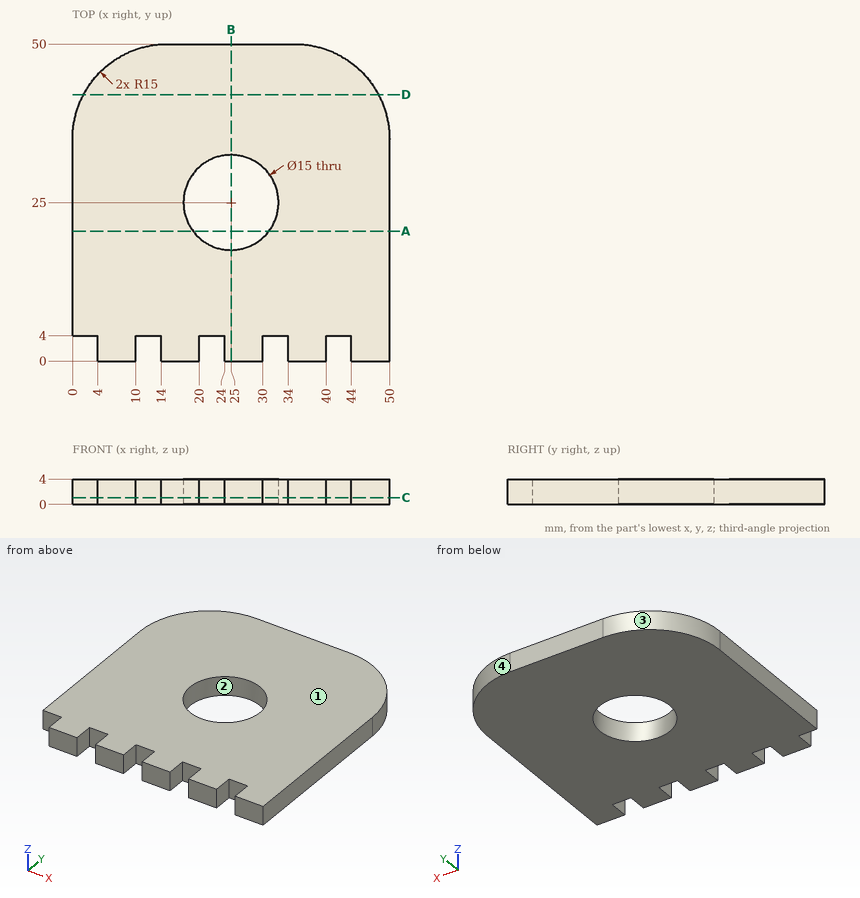
Can you work these out from the drawing? Everything is in mm from the part's minimum corner. Round coordinates to 2 decimals unless told otherwise and drop trailing zeros. Write each loop counter-clockwise with the first axis right and the second up, starting at its lowest first coordinate (ties: lowest second). Pieces come first, ordered by that corner, then holes. Notation, with made-up numbers: M 7,-13.5 L 50,-13.5 A21 cw 50,11.5 Z; hole C -4,63 d8. An arc over 180 degrees is marked long. Use a Markdown table: item, result.
Item 1: I want a section at D-D (y = 42). List the corners of the cut face in (x, z) for me.
Found:
| item | result |
|---|---|
| outline | M 1.73,0 L 48.27,0 L 48.27,4 L 1.73,4 Z |
Item 2: If I drill on line 1 along X through (y, z) = (2.5, 0.25); line 2 along Y through (x, z) = (25, 2.9); line 3 along Y through (x, z) = (22, 3.15), over which ranges is the centre line in solid material (lowest first)? Write a range as [from, to].
Found:
| item | result |
|---|---|
| line 1 | x = [4, 10], [14, 20], [24, 30], [34, 40], [44, 50] |
| line 2 | y = [0, 17.5], [32.5, 50] |
| line 3 | y = [4, 18.13], [31.87, 50] |
Item 3: I want a section at C-C (z = 1.05). List the corners of the cut face in (x, y) for me.
Found:
| item | result |
|---|---|
| outline | M 0,4 L 4,4 L 4,0 L 10,0 L 10,4 L 14,4 L 14,0 L 20,0 L 20,4 L 24,4 L 24,0 L 30,0 L 30,4 L 34,4 L 34,0 L 40,0 L 40,4 L 44,4 L 44,0 L 50,0 L 50,35 A15 ccw 35,50 L 15,50 A15 ccw 0,35 Z; hole C 25,25 d15 |
Item 4: For pin 1 Ø2 at (y, z) = (2.5, 2.5) entering from -X, with a flat end and sliding along its axis, tell me the tip position at first contact or that it passes through.
Found:
| item | result |
|---|---|
| pin 1 | stops at x = 4 |
Item 5: I want a section at A-A (y = 20.5). List the corners of the cut face in (x, z) for me.
Found:
| item | result |
|---|---|
| outline | M 0,0 L 19,0 L 19,4 L 0,4 Z; M 31,0 L 50,0 L 50,4 L 31,4 Z |
Item 6: I want a section at B-B (x = 25). List the corners of the cut face in (y, z) for me.
Found:
| item | result |
|---|---|
| outline | M 0,0 L 17.5,0 L 17.5,4 L 0,4 Z; M 32.5,0 L 50,0 L 50,4 L 32.5,4 Z |
Item 7: We'd pull the mould along X, two halves only. Please class the marked faces 1, 2, 3 and 4: released by +X, released by -X, zero draft, split by the parting line, or undercut.
Found:
| item | result |
|---|---|
| face 1 | zero draft |
| face 2 | undercut |
| face 3 | released by -X |
| face 4 | released by +X |
